from build123d import *

# Parameters (mm, degrees)
SKETCH1_R           = 106
BOSS_EXTRUDE1_DEPTH = 1
DOME1_FACE_RADIUS   = 106
DOME1_HEIGHT        = 68
SKETCH3_R           = 102.5
BOSS_EXTRUDE2_DEPTH = 1
DOME3_FACE_RADIUS   = 102.5
DOME3_HEIGHT        = 64
SKETCH4_R           = 141.495239339
CUT_EXTRUDE1_DEPTH  = 30
SKETCH6_W           = 177.061938601
SKETCH6_H           = 266.714694693
CUT_EXTRUDE3_DEPTH  = 61


with BuildPart() as part:
    # Sketch1 → Boss-Extrude1 (new body)
    with BuildSketch(Plane(origin=(0, 0, 0), x_dir=(1, 0, 0), z_dir=(0, 1, 0))):
        with Locations(Location((0, 0, 0), (0, 0, 270))):
            Circle(SKETCH1_R)
    extrude(amount=BOSS_EXTRUDE1_DEPTH)

    # Dome1: a dome of height H over a round flat face of radius A is a cap of a sphere of radius (A * A + H * H) / (2 * H)
    dome1_r = (DOME1_FACE_RADIUS * DOME1_FACE_RADIUS + DOME1_HEIGHT * DOME1_HEIGHT) / (2 * DOME1_HEIGHT)
    dome1_base = Plane((0, 1, 0), z_dir=(0, 1, 0))
    with Locations(dome1_base.offset(DOME1_HEIGHT - dome1_r)):
        dome1_ball = Sphere(dome1_r, mode=Mode.PRIVATE)
    add(split(dome1_ball, bisect_by=dome1_base, keep=Keep.TOP, mode=Mode.PRIVATE))

    # Sketch3 → Boss-Extrude2 (add)
    with BuildSketch(Plane.XZ):
        with Locations(Location((0, 0, 0), (0, 0, 270))):
            Circle(SKETCH3_R)
    extrude(amount=BOSS_EXTRUDE2_DEPTH)

    # Dome3: a dome of height H over a round flat face of radius A is a cap of a sphere of radius (A * A + H * H) / (2 * H)
    dome3_r = (DOME3_FACE_RADIUS * DOME3_FACE_RADIUS + DOME3_HEIGHT * DOME3_HEIGHT) / (2 * DOME3_HEIGHT)
    dome3_base = Plane((0, -1, 0), z_dir=(0, 1, 0))
    with Locations(dome3_base.offset(DOME3_HEIGHT - dome3_r)):
        dome3_ball = Sphere(dome3_r, mode=Mode.PRIVATE)
    add(split(dome3_ball, bisect_by=dome3_base, keep=Keep.TOP, mode=Mode.PRIVATE), mode=Mode.SUBTRACT)

    # Sketch4 → Cut-Extrude1 (cut)
    with BuildSketch(Plane(origin=(0, 69, 0), x_dir=(1, 0, 0), z_dir=(0, 1, 0))):
        Circle(SKETCH4_R)
    extrude(amount=-CUT_EXTRUDE1_DEPTH, mode=Mode.SUBTRACT)

    # Sketch6 → Cut-Extrude3 (cut)
    with BuildSketch(Plane(origin=(0, 39, 0), x_dir=(1, 0, 0), z_dir=(0, 1, 0))):
        with Locations((28.391818017, 2.178811005)):
            Rectangle(SKETCH6_W, SKETCH6_H)
    extrude(amount=-CUT_EXTRUDE3_DEPTH, mode=Mode.SUBTRACT)


solid = part.part
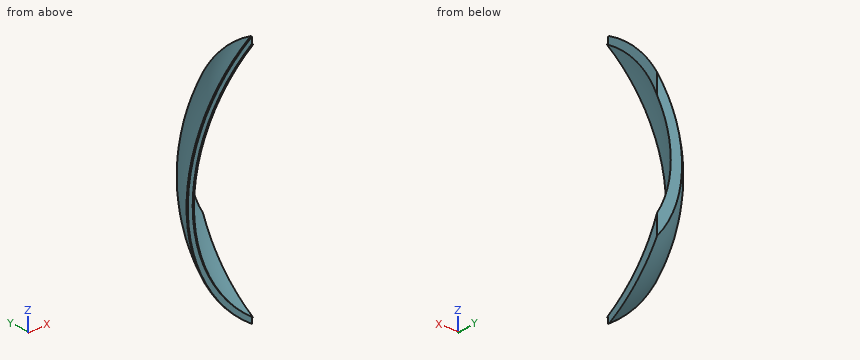
Source: CAD feature listing. Evaluate the final solid. Frame: model axes, mm. Coordinates: 2 decimals unless noted, no trailing zeros. Order: outer loops, then holes, each group sorted by start corner. A loop starts at its lowest first (then second) coordinate and runs counter-clockwise, first axis right, second up. Notation, with made-up numbers: M -37.5,44 L -12.5,44 A17 ccw -12.5,63 Z; hole C 32,-32 d4. An arc over 180 degrees is marked long. Write each question's results on one line, items separated by ' | '. Start each with the question number.
Item 1: Cut plane C-C (y = 25.5). Return loops of the section in (x, z), and give its area (3 significant figures).
Item 2: Cut plane D-D (z = 56). Return loops of the section in (x, y).
Item 3: Cut plane A-A (x = -90.5). Return loops of the section in (y, z), and give its area (3 significant figures).
Item 4: First-contact query: pin 1 Ø10 at (x, y) = (-84.5, 23) entering from +Z; pin 2 Ø12 at (y, z) = (3, -60) entering from -X; pin 3 Ø10 at (y, z) = (26, 52.5) entering from -X. Flat tips, straight axial feed; report the tip coordinate or a pass-through.
Item 5: Line query: probe 1 along Z at (x, y) = (-63, 21.5); probe 2 along Z at (x, y) = (-82.5, 15); probe 3 along X at (y, z) = (22.5, 12.5). Output: solid intervals per line, ascending.
Item 6: Cut plane B-B (z = -31). Return loops of the section in (x, y), and give its area (3 significant figures).
Checked values:
1) outline: M -60.14,-68.09 L -60.14,-59.44 A84.56 cw -60.14,59.44 L -60.14,68.09 A90.85 ccw Z | area: 900 mm2
2) outline: M -90,0 L -85.85,0 L -85.85,-1 A99.39 cw -60.14,28.05 L -60.14,35.13 A102.29 ccw -90,1 Z
3) outline: M -1,-48.12 L 0,-48.12 L 0,-55.19 L 1,-55.19 A73.55 ccw 1,55.19 L 0,55.19 L 0,48.12 L -1,48.12 A69.46 cw Z | area: 831 mm2
4) pin 1: stops at z = 50.49 | pin 2: stops at x = -91.01 | pin 3: stops at x = -79.39
5) probe 1: z = -69.67 to -61.46, 61.46 to 69.67 | probe 2: z = -53.6 to -42.91, 42.91 to 53.6 | probe 3: x = -92.34 to -86.28
6) outline: M -101.37,0 L -97.7,0 L -97.7,-1 A109.79 cw -62.76,39 L -71.67,39 A112.42 ccw -101.37,1 Z | area: 246 mm2
